Autodesk Inventor part; units mm, degrees
ref_plane "Plan de construction1" through (0, 0, 15.5) normal (0, 0, -1) x (-1, 0, 0)
ref_plane "YZ Plane" through (0, 0, 0) normal (1, 0, 0) x (0, 1, 0)
ref_plane "XZ Plane" through (0, 0, 0) normal (0, 1, 0) x (-1, 0, 0)
sketch "Esquisse1" plane through (0, 0, 0) normal (0, 0, 1) x (1, 0, 0)
  circle A0 centre (0, 0) radius 15
  line L0 (0, 0) -> (-10, 0)
  line L1 (0, 0) -> (0, 10)
  line L2 (0, 0) -> (10, 0)
  line L3 (0, 0) -> (0, -10)
  line L4 (0, -10) -> (10, 0)
  line L5 (10, 0) -> (0, 10)
  line L6 (0, 10) -> (-10, 0)
  line L7 (-10, 0) -> (0, -10)
  dimension "d0" = 30
  dimension "d1" = 10
  dimension "d2" = 10
  dimension "d3" = 10
  dimension "d4" = 10
extrude "Extrusion1" add sketch "Esquisse1" along normal blind 5.5
chamfer "Chanfrein1" distance 1 angle 45 1 edges at (-15, 0, 5.5)
sketch "Esquisse2" plane through (0, 0, 5.5) normal (0, 0, 1) x (1, 0, 0)
  circle A0 centre (0, 0) radius 11.5
  circle A1 centre (0, 0) radius 14
  line L0 (0, -10) -> (-10, 0)
  line L1 (0, 10) -> (10, 0)
  line L2 (-10, 0) -> (0, 10)
  line L3 (0, 10) -> (10, 0)
  line L4 (10, 0) -> (0, -10)
  line L5 (0, -10) -> (-10, 0)
  dimension "d10" = 23
  dimension "d26" = 28
extrude "Extrusion2" add sketch "Esquisse2" along normal blind 1 contours A0 | A1 | L0 L2 L1 L4
sketch "Esquisse3" plane through (0, 0, 6.5) normal (0, 0, 1) x (1, 0, 0)
  circle A0 centre (0, 0) radius 11
  circle A1 centre (0, 0) radius 14
  dimension "d13" = 22
  dimension "d27" = 28
extrude "Extrusion3" add sketch "Esquisse3" along normal blind 9
sketch "Esquisse4" plane through (0, 0, 6.5) normal (0, 0, 1) x (1, 0, 0)
  circle A0 centre (0, 0) radius 4.25
  dimension "d16" = 8.5
extrude "Extrusion4" cut sketch "Esquisse4" against normal through all
ref_plane "Plan de construction1" through (0, 0, 15.5) normal (0, 0, -1) x (-1, 0, 0)
sketch "Esquisse6" plane through (0, 0, 15.5) normal (0, 0, -1) x (-1, 0, 0)
  circle A0 centre (0, 0) radius 14
  line L0 (0, 0) -> (0, 12)
  line L1 (0, 12) -> (-1, 12)
  line L2 (-1, 12) -> (-1, 13.9642)
  circle A1 centre (0, 0) radius 14
  line L3 (0, 12) -> (1, 12)
  line L4 (1, 12) -> (1, 13.9642)
  dimension "d29" = 12
  dimension "d30" = 1
  dimension "d31" = 1
extrude "Extrusion6" cut sketch "Esquisse6" along normal blind 10 contours L4 L3 L1 L2 A0 picked at (-0.4445, 12.6653)
sketch "Esquisse7" plane through (0, 0, 6.5) normal (0, 0, 1) x (1, 0, 0)
  circle A0 centre (0, 0) radius 11
  circle A1 centre (0, 0) radius 7.5
  dimension "d34" = 15
extrude "Extrusion7" add sketch "Esquisse7" along normal blind 1
properties part number "bielle côté 2"
CAD build for the part. Positions are in the model's coordinates, mm. A direction names the side the tool comes from. Round coordinates to 2 decimals unless told otherwise and drop trailing zeros. Loops run counter-clockwise (first coordinate to the right, second up) from the corner with the lowest first, then second, coordinate; pieces in that order, holes last. Notation, with made-up numbers: M -5,26 L 33,26 A17 ccw 33,50 Z; hole C 58.25,87.5 d11. An arc over 180 degrees is marked long. One line per question, with ' | ' between items. Start each with the question number.
Item 1: Two-plate mould, pull along X, no slides. Class faces 1 (the cylindrical face through (-14.985, -0.66, 2.218)), 2 (the flat face through (3.2, -3.2, 6.5)), 3 (the flat face through (-4, 7, 0)): pulls with the +X half, pulls with the -X half, needs draft (parallel to the pull), parting line crosses it, or undercut.
Item 2: Cut at B-B, the plane z = 3.5. Write the cut outline in (x, y).
Item 3: Wall check: line 1 (Y direction, x = 0, z = 6.05); line 2 (Y direction, x = 0, z = 10); line 3 (Z direction, x = -5.5, y = 4.25). Give the ranges that are in metal, low to high.
Item 4: Pin check, flat tips, straight feed: pin 1 Ø7 at (x, y) = (0, 0) entering from -Z; pin 2 Ø4 at (x, z) = (7, 6) entering from -Y; pin 3 Ø1.5 at (y, z) = (-2.5, 7.5) entering from -X; pin 4 Ø0.6 at (y, z) = (13, 11) entering from +X. Stop position of each tip, or through.
Item 5: Which spindle directions (+Z, -Z, +X, -X, +Y, -Y) get a long thin tool onto all of the face, cutting with end or side? Do faces 4 (the flat face through (0, 12, 11)), 5 (the cylindrical face through (-7.493, -0.33, 6.993)), 6 (the flat face through (5, 5, 3)), 7 (the flat face through (-1.1, -11.3, 15.5)). Say none if no direction does.
Item 6: Cut at A-A, the plane z = 9.75. Write the cut outline in (x, y).
Responses:
1) face 1: parting line crosses it | face 2: undercut | face 3: needs draft
2) outline: C 0,0 d30; hole M -10,0 L 0,-10 L 10,0 L 0,10 Z
3) line 1: y = -14 to -4.25, 4.25 to 12 | line 2: y = -14 to -11, 11 to 12 | line 3: z = 5.5 to 6.5
4) pin 1: passes through | pin 2: stops at y = -13.88 | pin 3: stops at x = -13.89 | pin 4: stops at x = 5.89
5) face 4: +Z, +Y | face 5: +Z | face 6: -Z | face 7: +Z, +X, -X, +Y, -Y
6) outline: M -1,12 L -1,13.96 A14 ccw long 1,13.96 L 1,12 Z; hole C 0,0 d22
